Could you check a few things on this model? Use its own coordinates, in mm. Round coordinates to 2 decimals unless told otherwise and drop trailing zeros. Loops run counter-clockwise (first coordinate to the right, second up) from the corner with the lowest first, then second, coordinate; pieces in that order, holes last. Notation, with made-up numbers: (50, -3.5) -> (104, -3.5) arc R22 ccw to (104, 16.5) -> close; hole circle Ø3 at (58.5, 12.25). An arc over 180 degrees is marked (long way). One line per item, written item: value.
```python
from build123d import *

# Parameters (mm, degrees)
F0_W          = 50.8
F0_H          = 1.8034
F1_DEPTH      = 171.45
F1_DEPTH_BACK = 171.45
F2_W          = 25.4
F2_H          = 127
F3_DEPTH      = 1.8034
F5_DEPTH      = 1.8044


with BuildPart() as f1:
    # F0 (on Right) → F1 (new body, two sides)
    with BuildSketch(Plane.YZ) as f1_sk:
        Rectangle(F0_W, F0_H)
    extrude(amount=F1_DEPTH)
    extrude(f1_sk.sketch, amount=-F1_DEPTH_BACK)

    # F2 (on face) → F3 (join)
    with BuildSketch(Plane.XY.offset(0.9017)):
        with Locations((184.15, 38.1)):
            Rectangle(F2_W, F2_H)
    extrude(amount=-F3_DEPTH)

    # F4 (on face) → F5 (cut, through all)
    with BuildSketch(Plane.XY.offset(0.9017)):
        with BuildLine():
            ThreePointArc((-146.05, 13.81125), (-149.225, 10.63625), (-146.05, 7.46125))
            Line((-146.05, 7.46125), (133.35, 7.46125))
            ThreePointArc((133.35, 7.46125), (136.525, 10.63625), (133.35, 13.81125))
            Line((133.35, 13.81125), (-146.05, 13.81125))
        make_face()
    extrude(amount=-F5_DEPTH, mode=Mode.SUBTRACT)


solid = f1.part
```
Item 1: If we section it at B-B on z = -0.1: List the corners of the cut face in (x, y) for me (3 decimals), plus the area to 3 significant figures.
Output:
outline: (-171.45, -25.4) -> (196.85, -25.4) -> (196.85, 101.6) -> (171.45, 101.6) -> (171.45, 25.4) -> (-171.45, 25.4) -> close; hole (-146.05, 7.461) -> (133.35, 7.461) arc R3.175 ccw to (133.35, 13.811) -> (-146.05, 13.811) arc R3.175 ccw to start
area: 18,800 mm²
Item 2: Will these pins go through, and if not, where does the flat tip stop? pin 1 Ø0.9 at (y, z) = (80.5, 0.5) entering from -X; pin 2 Ø0.5 at (x, z) = (16.5, 0) entering from +Y.
Output:
pin 1: stops at x = 171.45
pin 2: stops at y = 25.4
Item 3: I need wall thicknesses on line 1 (Y direction, x = -58, z = -0.6); line 2 (X direction, y = 10.5, z = 0.55); line 3 (X direction, y = 78, z = -0.1). Which ranges of each line are inside material? Lowest first, please. Write a range as from..to.
Output:
line 1: y = -25.4..7.46, 13.81..25.4
line 2: x = -171.45..-149.22, 136.52..196.85
line 3: x = 171.45..196.85
Item 4: If we section it at C-C on y = 81: List the corners of the cut face in (x, z) for me.
Output:
outline: (171.45, -0.9) -> (196.85, -0.9) -> (196.85, 0.9) -> (171.45, 0.9) -> close
Item 5: If we section it at A-A on x = -86: List the corners of the cut face in (y, z) for me, plus the area to 3 significant figures.
Output:
outline: (-25.4, -0.9) -> (7.46, -0.9) -> (7.46, 0.9) -> (-25.4, 0.9) -> close; (13.81, -0.9) -> (25.4, -0.9) -> (25.4, 0.9) -> (13.81, 0.9) -> close
area: 80.2 mm²
